```python
from build123d import *

# Parameters (mm, degrees)
SKETCH_W     = 19
SKETCH_H     = 50.5
PAD_DEPTH    = 3.5
SKETCH001_R  = 1.5
SKETCH001_W  = 5.8
SKETCH001_H  = 12.6
POCKET_DEPTH = 3.5
FILLET_R     = 3
FILLET001_R  = 3
FILLET002_R  = 3
FILLET003_R  = 3


with BuildPart() as part:
    # Sketch → Pad (new body)
    with BuildSketch(Plane.XY):
        with Locations((7.5, 18.23)):
            Rectangle(SKETCH_W, SKETCH_H)
    extrude(amount=PAD_DEPTH)

    # Sketch001 (on Face6 of Pad) → Pocket (cut)
    with BuildSketch(Plane.XY.offset(3.5)):
        with Locations((7.5, -4)):
            Circle(SKETCH001_R)
        with Locations((7.5, 40.05)):
            Circle(SKETCH001_R)
        with Locations((2.9, 29.75)):
            Rectangle(SKETCH001_W, SKETCH001_H)
        with Locations((12.71, 29.75)):
            Rectangle(SKETCH001_W, SKETCH001_H)
        with Locations((2.9, 6.3)):
            Rectangle(SKETCH001_W, SKETCH001_H)
        with Locations((12.71, 6.3)):
            Rectangle(SKETCH001_W, SKETCH001_H)
    extrude(amount=-POCKET_DEPTH, mode=Mode.SUBTRACT)

    # Fillet
    fillet_edges = [part.edges().sort_by_distance(p)[0] for p in [
        (-2, 43.48, 1.75),
    ]]
    fillet(fillet_edges, radius=FILLET_R)

    # Fillet001
    fillet001_edges = [part.edges().sort_by_distance(p)[0] for p in [
        (17, 43.48, 1.75),
    ]]
    fillet(fillet001_edges, radius=FILLET001_R)

    # Fillet002
    fillet002_edges = [part.edges().sort_by_distance(p)[0] for p in [
        (17, -7.02, 1.75),
    ]]
    fillet(fillet002_edges, radius=FILLET002_R)

    # Fillet003
    fillet003_edges = [part.edges().sort_by_distance(p)[0] for p in [
        (-2, -7.02, 1.75),
    ]]
    fillet(fillet003_edges, radius=FILLET003_R)


solid = part.part
```
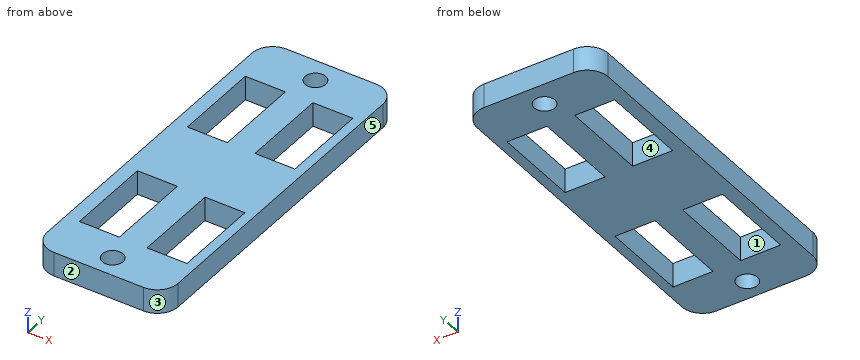
CAD build for the part. Positions are in the model's coordinates, mm. Face numbers are marked on the shaded views. A direction names the side the tool comes from. Give positions to 0.01 mm unless a question says otherwise; leave off trailing zeros. Order: outer loops, then holes, each group sorted by start corner. A loop starts at its lowest first (then second) coordinate and runs counter-clockwise, first axis right, second up. Notation, with made-up numbers: M 27,22.25 L 31,22.25 A12 ccw 31,28.25 Z; hole C -32,70 d9. An arc over 180 degrees is marked long. Put each result on its own line as item: value. Start each with the question number.
(1) Mould opens along X. For the marked faces 1, 2 and 3 say: +X half, -X half, draft (parallel to the pull), parting line (faces both ways), or undercut.
(2) Drill centre lines: line 1 along Y through (x, z) = (7.5, 2.55); line 2 along X through (y, z) = (30.5, 1.7); line 3 along Y through (x, z) = (4.75, 1.05). Where is each one in solid material? Low to high.
(3) Which spindle directions (+Z, -Z, +X, -X, +Y, -Y) get a long thin tool onto all of the face, cutting with end or side? Do the marked faces 4 and 5. Say none if no direction does.
(4) Saw through at B-B, the plane z = 2.5. Write the cut outline in (x, y), then the cut area to 3 significant figures.
(5) Saw through at A-A, the plane x = 7.5. Write the cut outline in (y, z), then the cut area to 3 significant figures.
(6) Flat gauge pin, fed straight in: pin 1 Ø4 at (x, y) = (11.5, 32.5) entering from -Z. Where does the tip first touch, or does it go through?
(7) Saw through at C-C, the plane x = 12.25. Write the cut outline in (y, z), then the cut area to 4 significant figures.
Check result:
1. face 1: undercut
1. face 2: draft
1. face 3: +X half
2. line 1: y = -7.02 to -5.5, -2.5 to 38.55, 41.55 to 43.48
2. line 2: x = -2 to 0, 5.8 to 9.81, 15.61 to 17
2. line 3: y = -7.02 to 0, 12.6 to 23.45, 36.05 to 43.48
3. face 4: +Z, -Z
3. face 5: +Z, -Z, +X, +Y, -Y
4. outline: M -2,-4.02 A3 ccw 1,-7.02 L 14,-7.02 A3 ccw 17,-4.02 L 17,40.48 A3 ccw 14,43.48 L 1,43.48 A3 ccw -2,40.48 Z; hole M 0,0 L 5.8,0 L 5.8,12.6 L 0,12.6 Z; hole M 0,23.45 L 5.8,23.45 L 5.8,36.05 L 0,36.05 Z; hole C 7.5,-4 d3; hole C 7.5,40.05 d3; hole M 9.81,0 L 15.61,0 L 15.61,12.6 L 9.81,12.6 Z; hole M 9.81,23.45 L 15.61,23.45 L 15.61,36.05 L 9.81,36.05 Z
4. area: 645 mm2
5. outline: M -7.02,0 L -5.5,0 L -5.5,3.5 L -7.02,3.5 Z; M -2.5,0 L 38.55,0 L 38.55,3.5 L -2.5,3.5 Z; M 41.55,0 L 43.48,0 L 43.48,3.5 L 41.55,3.5 Z
5. area: 156 mm2
6. pin 1: stops at z = 0
7. outline: M -7.02,0 L 0,0 L 0,3.5 L -7.02,3.5 Z; M 12.6,0 L 23.45,0 L 23.45,3.5 L 12.6,3.5 Z; M 36.05,0 L 43.48,0 L 43.48,3.5 L 36.05,3.5 Z
7. area: 88.55 mm2
